from build123d import *

# Parameters (mm, degrees)
BOSS_EXTRUDE1_DEPTH = 5
SKETCH2_R           = 77.5
BOSS_EXTRUDE2_DEPTH = 5
CUT_EXTRUDE1_DEPTH  = 6


with BuildPart() as part:
    # Sketch1 → Boss-Extrude1 (new body)
    with BuildSketch(Plane(origin=(0, 0, 0), x_dir=(1, 0, 0), z_dir=(0, 1, 0))):
        with BuildLine():
            Line((107.884615385, 10.824036369), (57.115384615, 59.532200029))
            ThreePointArc((57.115384615, 59.532200029), (0, 82.5), (-57.115384615, 59.532200029))
            Line((-57.115384615, 59.532200029), (-107.884615385, 10.824036369))
            ThreePointArc((-107.884615385, 10.824036369), (-112.5, 0), (-107.884615385, -10.824036369))
            Line((-107.884615385, -10.824036369), (-57.115384615, -59.532200029))
            ThreePointArc((-57.115384615, -59.532200029), (0, -82.5), (57.115384615, -59.532200029))
            Line((57.115384615, -59.532200029), (107.884615385, -10.824036369))
            ThreePointArc((107.884615385, -10.824036369), (112.5, 0), (107.884615385, 10.824036369))
        make_face()
    extrude(amount=BOSS_EXTRUDE1_DEPTH)

    # Sketch2 → Boss-Extrude2 (add)
    with BuildSketch(Plane(origin=(0, 5, 0), x_dir=(1, 0, 0), z_dir=(0, 1, 0))):
        Circle(SKETCH2_R)
    extrude(amount=BOSS_EXTRUDE2_DEPTH)

    # Sketch3 → Cut-Extrude1 (cut, through all)
    with BuildSketch(Plane(origin=(0, 5, 0), x_dir=(1, 0, 0), z_dir=(0, 1, 0))):
        Polygon((-95.190598923, 4), (-99.809401077, 4), (-102.118802154, 0), (-99.809401077, -4), (-95.190598923, -4), (-92.881197846, 0), align=None)
        Polygon((99.809401077, 4), (95.190598923, 4), (92.881197846, 0), (95.190598923, -4), (99.809401077, -4), (102.118802154, 0), align=None)
    extrude(amount=-CUT_EXTRUDE1_DEPTH, mode=Mode.SUBTRACT)


solid = part.part
Geometry check sheet. Reference: the model listing, model coordinates, mm. A direction names the side the tool comes from. Round coordinates to 2 decimals unless told otherwise and drop trailing zeros. Loops run counter-clockwise (first coordinate to the right, second up) from the corner with the lowest first, then second, coordinate; pieces in that order, holes last.
Item 1: Cross-section at C-C on z = -42. Record the boundary of the cut face in (x, y), then the cut area to 3 significant figures.
Item 2: Access from +Z, -Z, +X, -X, +Y, -Y to the whole of each face (thin tool, end or side, straight path). Record for faces 1 (the flat face through (-97, 3, -4)), 2 (the flat face through (82.145, 2.465, 35.519)), 3 (the flat face through (24, 5, -74)).
Item 3: Gauge pin test, flat ends, axial feed: pin 1 (6 mm diameter, centred on y = 1, z = 39, fed in from -X); pin 2 (6 mm diameter, centred on y = 4.5, z = -20, fed in from +X); pin 3 (2.5 mm diameter, centred on x = 97.5, y = 3.5, fed in from +Z). Record the tip position at first contact, or that the pin passes through.
Item 4: Mould release check, pull along Z, two halves, no side actions. Record for faces 4 (the cylindrical face through (-0.883, 2.465, 82.495)), 5 (the flat face through (-98, 3, 4)), 6 (the cylindrical face through (0.883, 2.465, -82.495)): pulls with the +Z half, pulls with the -Z half, needs draft (parallel to the pull), parting line crosses it, or undercut.
Item 5: Cross-section at D-D on x = -80.5. Record the boundary of the cut face in (y, z).
Item 6: Cross-section at A-A on y = 3.25. Record the boundary of the cut face in (x, z), then the cut area to 3 significant figures.
Item 7: Cross-section at B-B on x = 0. Record the boundary of the cut face in (y, z).
Item 8: Thickness scan on line 1 (Y direction, x = -79.5, z = -8); line 2 (Z direction, x = -101.5, y = 4.75); line 3 (X direction, y = 4.75, z = 49.5). Record the ranges inside material, lowest first.
Answer sheet:
1. outline: (-75.39, 0) - (75.39, 0) - (75.39, 5) - (65.13, 5) - (65.13, 10) - (-65.13, 10) - (-65.13, 5) - (-75.39, 5) - close
1. area: 1,410 mm2
2. face 1: +Y, -Y
2. face 2: +Z, +X, +Y, -Y
2. face 3: +Y
3. pin 1: stops at x = -81.64
3. pin 2: stops at x = 101.45
3. pin 3: stops at z = 21.99
4. face 4: pulls with the +Z half
4. face 5: undercut
4. face 6: pulls with the -Z half
5. outline: (0, -37.1) - (5, -37.1) - (5, 37.1) - (0, 37.1) - close
6. outline: (-107.88, -10.82) - (-57.12, -59.53) arc R82.5 ccw to (57.12, -59.53) - (107.88, -10.82) arc R15 ccw to (107.88, 10.82) - (57.12, 59.53) arc R82.5 ccw to (-57.12, 59.53) - (-107.88, 10.82) arc R15 ccw to start; hole (-102.12, 0) - (-99.81, -4) - (-95.19, -4) - (-92.88, 0) - (-95.19, 4) - (-99.81, 4) - close; hole (92.88, 0) - (95.19, -4) - (99.81, -4) - (102.12, 0) - (99.81, 4) - (95.19, 4) - close
6. area: 24,400 mm2
7. outline: (0, -82.5) - (5, -82.5) - (5, -77.5) - (10, -77.5) - (10, 77.5) - (5, 77.5) - (5, 82.5) - (0, 82.5) - close
8. line 1: y = 0 to 5
8. line 2: z = -16.95 to -1.07, 1.07 to 16.95
8. line 3: x = -67.57 to 67.57
